Study the drawing (mm; zero at the part's minimum x, y, z) and answer. A direction names the side the tool comes from. Round coordinates to 2 decimals unless told otherwise and drop trailing zeros. Order: outer loops, then holes, each group sorted by start corner. A loop starts at its lowest first (then second) coordinate and runs counter-clockwise, first axis right, second up. Notation, with made-up numbers: (23.5, -23) - (54.5, -23) arc R24 cw to (54.5, 14) - close; hole circle Ø2 at (6, -33.75). An arc over 180 degrees is marked (long way). Use one line per item in the form item = value. Start each with the question number.
Q1. The part is cut by section A-A on y = 20. Determine the outline of the cut face in (x, z), plus the area to 3 significant figures.
Q2. The part is cut by section C-C on z = 20.5. Determine the outline of the cut face in (x, y).
Q3. The part is cut by section D-D on y = 29. Determine the outline of the cut face in (x, z), plus the area to 3 significant figures.
Q4. Which of the six approach directions +Z, -Z, +X, -X, +Y, -Y give full straight-line access (tool end or side, diameter ignored) to the marked faces 1, 2 and 3?
Q5. For a pull along Y with two mould halves and no side action, classify the marked faces 4, 5, 6 and 7 as +Y half, -Y half, draft (parallel to the pull), parting line (faces both ways), or undercut.
Q6. Find the intervals of material crossed by line 1 (X direction, y = 19, z = 16); line 2 (Z direction, x = 4.5, y = 8.5); line 3 (X direction, y = 32, z = 15), in increasing order. Write a range as [from, to].
Q7. The part is cut by section B-B on x = 15.5. Determine the outline of the cut face in (y, z).
Q8. Given P1, Ø12, axis at x = 20.5, y = 32.5, coming from the +Z side; P2, Ø12, axis at x = 34, y = 8.5, coming from the -Z side; P3, Ø4, axis at x = 42, y = 28, coming from the +Z side; P4, Ø11, axis at y = 22, z = 7.5, coming from the -X side, each flat-ended and moving along its own axis, determine where each tip first touches the part or whether it passes through.
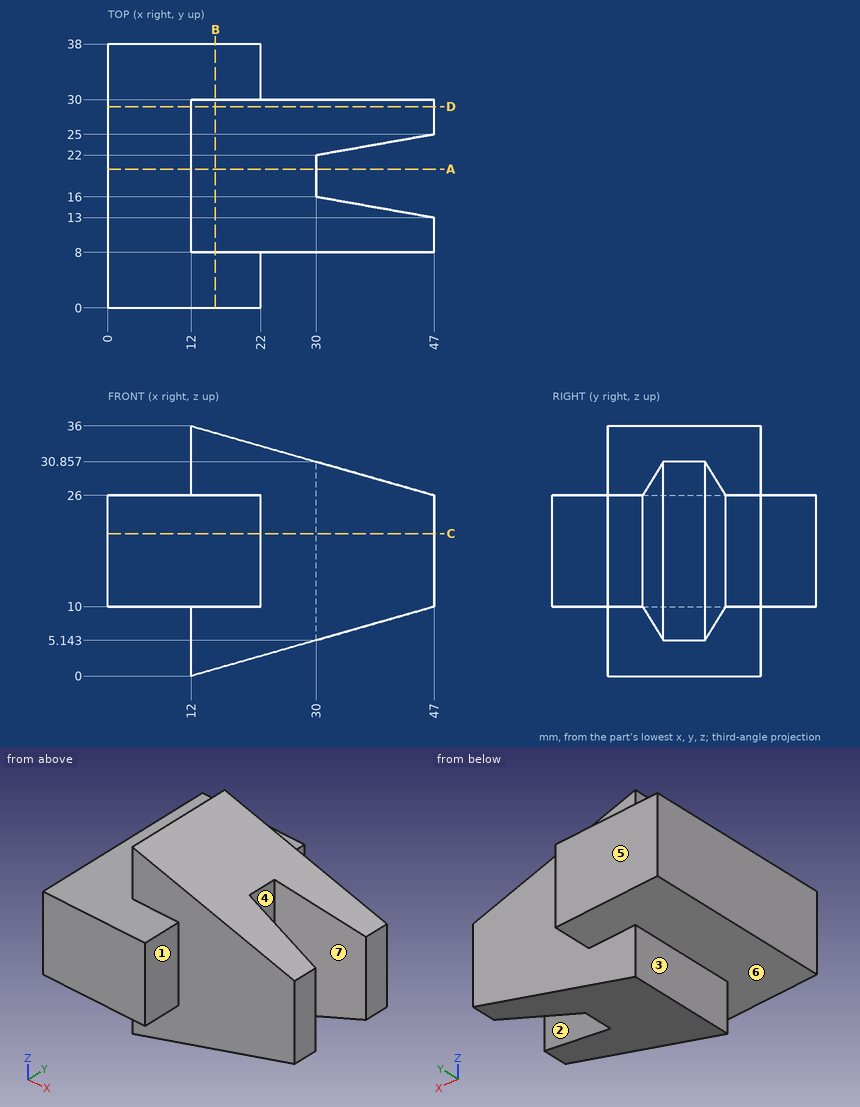
Found:
q1.outline = (0, 10) - (12, 10) - (12, 0) - (30, 5.14) - (30, 30.86) - (12, 36) - (12, 26) - (0, 26) - close
q1.area = 747 mm²
q2.outline = (0, 0) - (22, 0) - (22, 8) - (47, 8) - (47, 13) - (30, 16) - (30, 22) - (47, 25) - (47, 30) - (22, 30) - (22, 38) - (0, 38) - close
q3.outline = (0, 10) - (12, 10) - (12, 0) - (47, 10) - (47, 26) - (12, 36) - (12, 26) - (0, 26) - close
q3.area = 1,100 mm²
q4.face_1 = +Z, -Z, +X, -Y
q4.face_2 = +Z, -Z, +X
q4.face_3 = -Z, -X, +Y, -Y
q5.face_4 = undercut
q5.face_5 = +Y half
q5.face_6 = draft
q5.face_7 = undercut
q6.line_1 = [0, 30]
q6.line_2 = [10, 26]
q6.line_3 = [0, 22]
q7.outline = (0, 10) - (8, 10) - (8, 1) - (30, 1) - (30, 10) - (38, 10) - (38, 26) - (30, 26) - (30, 35) - (8, 35) - (8, 26) - (0, 26) - close
q8.P1 = 35.13
q8.P2 = 4.57
q8.P3 = 28
q8.P4 = 0
